```python
from build123d import *

# Parameters (mm, degrees)
SKETCH1_R                       = 3.5
BOSS_EXTRUDE1_DEPTH             = 11
BOSS_EXTRUDE1_2_DEPTH           = 11
BOSS_EXTRUDE1_3_DEPTH           = 11
BOSS_EXTRUDE1_4_DEPTH           = 11
BOSS_EXTRUDE2_START             = -1
BOSS_EXTRUDE2_DEPTH             = 1
F_4_0MM_DOWEL_HOLE1_D           = 4
BOSS_EXTRUDE3_START             = 3
BOSS_EXTRUDE3_DEPTH             = 3
BOSS_EXTRUDE4_REACH             = 64.845
SKETCH11_W                      = 7
SKETCH11_H                      = 7
BOSS_EXTRUDE4_DIRECTION_2_DEPTH = 1
FILLET1_R                       = 2
M3_CLEARANCE_HOLE1_D            = 3.6
SKETCH15_R                      = 4.3
CUT_EXTRUDE1_DEPTH              = 5
BOSS_EXTRUDE6_START             = -1
BOSS_EXTRUDE6_DEPTH             = 5.5


with BuildPart() as part:
    # Sketch1 → Boss-Extrude1 (new body)
    with BuildSketch(Plane(origin=(0, 0, 0), x_dir=(1, 0, 0), z_dir=(0, 1, 0))):
        with Locations(Location((0, 51, 0), (0, 0, 270))):
            Circle(SKETCH1_R)
    extrude(amount=BOSS_EXTRUDE1_DEPTH)



with BuildPart() as body_2:
    # Sketch1 → Boss-Extrude1 2 (new body)
    with BuildSketch(Plane(origin=(0, 0, 0), x_dir=(1, 0, 0), z_dir=(0, 1, 0))):
        with Locations(Location((27, 51, 0), (0, 0, 270))):
            Circle(SKETCH1_R)
    extrude(amount=BOSS_EXTRUDE1_2_DEPTH)


with BuildPart() as body_3:
    # Sketch1 → Boss-Extrude1 3 (new body)
    with BuildSketch(Plane(origin=(0, 0, 0), x_dir=(1, 0, 0), z_dir=(0, 1, 0))):
        with Locations(Location((27, 0, 0), (0, 0, 270))):
            Circle(SKETCH1_R)
    extrude(amount=BOSS_EXTRUDE1_3_DEPTH)


with BuildPart() as body_4:
    # Sketch1 → Boss-Extrude1 4 (new body)
    with BuildSketch(Plane(origin=(0, 0, 0), x_dir=(1, 0, 0), z_dir=(0, 1, 0))):
        with Locations(Location((0, 0, 0), (0, 0, 270))):
            Circle(SKETCH1_R)
    extrude(amount=BOSS_EXTRUDE1_4_DEPTH)


with BuildPart() as part_1:
    add(part.part)

    add(body_2.part)  # Boss-Extrude2 merges body 2

    add(body_3.part)  # Boss-Extrude2 merges body 3

    add(body_4.part)  # Boss-Extrude2 merges body 4
    # Sketch2 → Boss-Extrude2 (add)
    with BuildSketch(Plane(origin=(0, 11, 0), x_dir=(1, 0, 0), z_dir=(0, 1, 0)).offset(BOSS_EXTRUDE2_START)):
        with BuildLine():
            Line((27, 54.5), (0, 54.5))
            ThreePointArc((0, 54.5), (-2.474873734, 53.474873734), (-3.5, 51))
            Line((-3.5, 51), (-3.5, 0))
            ThreePointArc((-3.5, 0), (-2.474873734, -2.474873734), (0, -3.5))
            Line((0, -3.5), (27, -3.5))
            ThreePointArc((27, -3.5), (29.474873734, -2.474873734), (30.5, 0))
            Line((30.5, 0), (30.5, 51))
            ThreePointArc((30.5, 51), (29.474873734, 53.474873734), (27, 54.5))
        make_face()
    extrude(amount=BOSS_EXTRUDE2_DEPTH)

    # Ø4.0mm Dowel Hole1 (through all)
    with Locations(Plane(origin=(0, 0, 0), x_dir=(-1, 0, 0), z_dir=(0, -1, 0))):
        with Locations((-27, 51), (0, 51), (0, 0), (-27, 0)):
            Hole(F_4_0MM_DOWEL_HOLE1_D / 2)

    # Sketch10 → Boss-Extrude3 (add)
    with BuildSketch(Plane.XZ.offset(-10).offset(BOSS_EXTRUDE3_START)):
        with BuildLine():
            ThreePointArc((-3.5, -51), (-2.958039892, -49.129171307), (-1.5, -47.83772234))
            Line((-1.5, -47.83772234), (-1.5, -3.16227766))
            ThreePointArc((-1.5, -3.16227766), (-2.958039892, -1.870828693), (-3.5, 0))
            Line((-3.5, 0), (-3.5, -51))
        make_face()
        with BuildLine():
            Line((3.16227766, 1.5), (23.83772234, 1.5))
            ThreePointArc((23.83772234, 1.5), (25.129171307, 2.958039892), (27, 3.5))
            Line((27, 3.5), (0, 3.5))
            ThreePointArc((0, 3.5), (1.870828693, 2.958039892), (3.16227766, 1.5))
        make_face()
        with BuildLine():
            Line((12.36850682, -25.5), (13.5, -23.362735104))
            Line((13.5, -23.362735104), (2.453131039, -2.496427068))
            ThreePointArc((2.453131039, -2.496427068), (1.637607021, -3.093257707), (0.685555207, -3.432202508))
            Line((0.685555207, -3.432202508), (12.36850682, -25.5))
        make_face()
        with BuildLine():
            ThreePointArc((26.314444793, -3.432202508), (25.362392979, -3.093257707), (24.546868961, -2.496427068))
            Line((24.546868961, -2.496427068), (13.5, -23.362735104))
            Line((13.5, -23.362735104), (14.63149318, -25.5))
            Line((14.63149318, -25.5), (26.314444793, -3.432202508))
        make_face()
        with BuildLine():
            ThreePointArc((30.5, 0), (29.958039892, -1.870828693), (28.5, -3.16227766))
            Line((28.5, -3.16227766), (28.5, -47.83772234))
            ThreePointArc((28.5, -47.83772234), (29.958039892, -49.129171307), (30.5, -51))
            Line((30.5, -51), (30.5, 0))
        make_face()
        with BuildLine():
            ThreePointArc((27, -54.5), (25.129171307, -53.958039892), (23.83772234, -52.5))
            Line((23.83772234, -52.5), (3.16227766, -52.5))
            ThreePointArc((3.16227766, -52.5), (1.870828693, -53.958039892), (0, -54.5))
            Line((0, -54.5), (27, -54.5))
        make_face()
        Polygon((14.63149318, -25.5), (13.5, -23.362735104), (12.36850682, -25.5), (13.5, -27.637264896), align=None)
        with BuildLine():
            Line((26.314444793, -47.567797492), (14.63149318, -25.5))
            Line((14.63149318, -25.5), (13.5, -27.637264896))
            Line((13.5, -27.637264896), (24.546868961, -48.503572932))
            ThreePointArc((24.546868961, -48.503572932), (25.362392979, -47.906742293), (26.314444793, -47.567797492))
        make_face()
        with BuildLine():
            Line((13.5, -27.637264896), (12.36850682, -25.5))
            Line((12.36850682, -25.5), (0.685555207, -47.567797492))
            ThreePointArc((0.685555207, -47.567797492), (1.637607021, -47.906742293), (2.453131039, -48.503572932))
            Line((2.453131039, -48.503572932), (13.5, -27.637264896))
        make_face()
    extrude(amount=-BOSS_EXTRUDE3_DEPTH)

    # Boss-Extrude4: up to this face of the body (flat: up to its plane)
    boss_extrude4_end = Plane(part_1.part.faces().sort_by_distance((13.5, 11, -25.5))[0])
    # Sketch11 → Boss-Extrude4 (add, up to the picked face)
    with BuildSketch(Plane.XZ.offset(-7), mode=Mode.PRIVATE) as boss_extrude4_sk1:
        with Locations((34, -12)):
            Rectangle(SKETCH11_W, SKETCH11_H)
    boss_extrude4_tool1 = split(extrude(boss_extrude4_sk1.sketch, amount=-BOSS_EXTRUDE4_REACH, mode=Mode.PRIVATE), bisect_by=boss_extrude4_end, keep=Keep.BOTH, mode=Mode.PRIVATE)
    # Sketch11 → Boss-Extrude4 (add, up to the picked face)
    with BuildSketch(Plane.XZ.offset(-7), mode=Mode.PRIVATE) as boss_extrude4_sk2:
        with Locations((34, -39)):
            Rectangle(SKETCH11_W, SKETCH11_H)
    boss_extrude4_tool2 = split(extrude(boss_extrude4_sk2.sketch, amount=-BOSS_EXTRUDE4_REACH, mode=Mode.PRIVATE), bisect_by=boss_extrude4_end, keep=Keep.BOTH, mode=Mode.PRIVATE)
    add(boss_extrude4_tool1.solids().sort_by(Axis((34, 7, -12), (0, 1, 0)))[0])
    add(boss_extrude4_tool2.solids().sort_by(Axis((34, 7, -39), (0, 1, 0)))[0])

    # Sketch11 → Boss-Extrude4 direction 2 (add)
    with BuildSketch(Plane.XZ.offset(-7)):
        with Locations((34, -12)):
            Rectangle(SKETCH11_W, SKETCH11_H)
        with Locations((34, -39)):
            Rectangle(SKETCH11_W, SKETCH11_H)
    extrude(amount=BOSS_EXTRUDE4_DIRECTION_2_DEPTH)

    # Fillet1
    fillet1_edges = [part_1.edges().sort_by_distance(p)[0] for p in [
        (30.5, 9, -15.5),
        (37.5, 8.5, -15.5),
        (37.5, 8.5, -8.5),
        (30.5, 9, -35.5),
        (37.5, 8.5, -42.5),
        (37.5, 8.5, -35.5),
    ]]
    fillet(fillet1_edges, radius=FILLET1_R)

    # M3 Clearance Hole1 (through all)
    with Locations(Plane(origin=(0, 6, 0), x_dir=(-1, 0, 0), z_dir=(0, -1, 0))):
        with Locations((-34, 12), (-34, 39)):
            Hole(M3_CLEARANCE_HOLE1_D / 2)

    # Sketch15 → Cut-Extrude1 (cut)
    with BuildSketch(Plane(origin=(0, 11, 0), x_dir=(1, 0, 0), z_dir=(0, 1, 0))):
        with Locations((2.5, 48.5)):
            Circle(SKETCH15_R)
        with Locations((2.5, 2.5)):
            Circle(SKETCH15_R)
    extrude(amount=-CUT_EXTRUDE1_DEPTH, mode=Mode.SUBTRACT)

    # Sketch17 → Boss-Extrude6 (add)
    with BuildSketch(Plane.XZ.offset(-10).offset(BOSS_EXTRUDE6_START)):
        with BuildLine():
            Line((2.5, 1.8), (2.5, 3.8))
            ThreePointArc((2.5, 3.8), (6.954772721, -6.954772721), (-3.8, -2.5))
            Line((-3.8, -2.5), (-1.8, -2.5))
            ThreePointArc((-1.8, -2.5), (5.540559159, -5.540559159), (2.5, 1.8))
        make_face()
        with BuildLine():
            Line((-1.8, -48.5), (-3.8, -48.5))
            ThreePointArc((-3.8, -48.5), (6.954772721, -44.045227279), (2.5, -54.8))
            Line((2.5, -54.8), (2.5, -52.8))
            ThreePointArc((2.5, -52.8), (5.540559159, -45.459440841), (-1.8, -48.5))
        make_face()
    extrude(amount=BOSS_EXTRUDE6_DEPTH)


solid = part_1.part
```
For this review, take the finished solid that the model builds, in its own axes (mm). A direction names the side the tool comes from. Round coordinates to 2 decimals unless told otherwise and drop trailing zeros. Write each loop counter-clockwise with the first axis right and the second up, starting at its lowest first coordinate (ties: lowest second). Pieces come first, ordered by that corner, then holes. Notation, with made-up numbers: (88.25, 4.5) -> (143.25, 4.5) arc R30 cw to (143.25, 38.5) -> close; hole circle Ø6 at (-22.5, 79.25). An arc over 180 degrees is marked (long way). Use one line per item in the form item = value.
1) Clearance check with flat-ended pins moving along their axes: pin 1 (5.5 mm diameter, centred on x = 32.5, z = -12, fed in from -Y); pin 2 (4.5 mm diameter, centred on y = 10, z = -48.5, fed in from +X); pin 3 (15.5 mm diameter, centred on x = 19.5, z = -16.5, fed in from -Y). State where each tip first meets the part, or that it passes through.
Found:
pin_1 = 6
pin_2 = 30.5
pin_3 = 7
2) Take a section at A-A, the plane y = 3.75. Write out the cut boundary in (x, z).
Found:
outline = circle Ø7 at (0, -51); circle Ø7 at (0, 0); circle Ø7 at (27, -51); circle Ø7 at (27, 0); hole circle Ø4 at (0, -51); hole circle Ø4 at (0, 0); hole circle Ø4 at (27, -51); hole circle Ø4 at (27, 0)
3) To check wall thickness, follow L1, parallel to Z at x = 34, y = 9.45; L2, parallel to Z at x = 27, y = 3.75; L3, parallel to X at y = 8, z = -17.5. State the ranges of each line that lie inside material, in increasing order. Write a range as from..to.
Found:
L1 = -42.5..-40.8, -37.2..-35.5, -15.5..-13.8, -10.2..-8.5
L2 = -54.5..-53, -49..-47.5, -3.5..-2, 2..3.5
L3 = -3.5..-1.5, 8.13..10.4, 16.6..18.87, 28.5..30.5
4) Take a section at D-D, the plane y = 8.5. Count the separate pieces of the cut face and the enclosed holes in it, and give its area (3 significant figures).
Found:
separate_pieces = 1
enclosed_holes = 10
area = 676 mm2
5) Tool access review of faces 5 (the cylindrical face through (31.07, 9.03, -16.1)), 6 (the flat face through (7.865, 8.479, -16.994)), 7 (the flat face through (-3.5, 9, -25)): name each direction out of +Z, -Z, +X, -X, +Y, -Y from which nothing blocks a thin tool from reaching the whole face with its end or side.
Found:
face_5 = +X, +Y, -Y
face_6 = -Y
face_7 = -X, +Y, -Y
6) Mouldability with a two-part tool opening along Z and no side actions: class faces 1 (the flat face through (16, 9, -54.5)), 2 (the flat face through (17, 11, -26)), 3 (the flat face through (30, 7, -25)), 4 (the flat face through (9.4, 8.48, -35.38)) as +Z half, -Z half, draft (parallel to the pull), parting line (faces both ways), or undercut.
Found:
face_1 = -Z half
face_2 = draft
face_3 = undercut
face_4 = undercut
7) Take a section at C-C, the plane x = 18. Write out the cut boundary in (y, z).
Found:
outline = (7, -54.5) -> (11, -54.5) -> (11, 3.5) -> (7, 3.5) -> (7, 1.5) -> (10, 1.5) -> (10, -14.86) -> (7, -14.86) -> (7, -19.14) -> (10, -19.14) -> (10, -31.86) -> (7, -31.86) -> (7, -36.14) -> (10, -36.14) -> (10, -52.5) -> (7, -52.5) -> close
8) Take a section at B-B, the plane z = -39. Write out the cut boundary in (x, y).
Found:
outline = (-3.5, 7) -> (-1.5, 7) -> (-1.5, 10) -> (5.22, 10) -> (5.22, 7) -> (7.48, 7) -> (7.48, 10) -> (19.52, 10) -> (19.52, 7) -> (21.78, 7) -> (21.78, 10) -> (28.5, 10) -> (28.5, 7) -> (30.5, 7) -> (30.5, 6) -> (32.2, 6) -> (32.2, 11) -> (-3.5, 11) -> close; (35.8, 6) -> (37.5, 6) -> (37.5, 11) -> (35.8, 11) -> close
